from build123d import *

# Parameters (mm, degrees)
SKETCH_2_R = 0.5


with BuildPart() as part:
    # 扫描1: sweep along a path in 草图1
    with BuildLine(Plane.XY) as sweep_1_path:
        Line((-0.5, 0), (-4, 0))
        Line((-4, 0), (-4, 2))
        ThreePointArc((-4, 2), (0, 6), (4, 2))
        Line((4, 2), (4, 0))
        Line((4, 0), (0.5, 0))
    # 草图2 → 扫描1 (sweep)
    with BuildSketch(Plane(origin=(-0.5, 0, 0), x_dir=(0, 0, -1), z_dir=(1, 0, 0))):
        Circle(SKETCH_2_R)
    sweep(path=sweep_1_path.line, transition=Transition.RIGHT)


solid = part.part
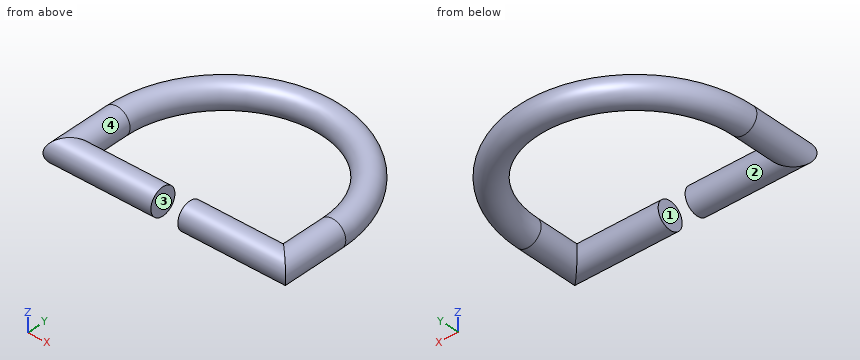
CAD build for the part. Positions are in the model's coordinates, mm. Face numbers are marked on the shaded views. A direction names the side the tool comes from. Coordinates: 2 decimals unless noted, no trailing zeros. Order: outer loops, then holes, each group sorted by start corner. A loop starts at its lowest first (then second) coordinate and runs counter-clockwise, first axis right, second up.
Item 1: 3-axis set-ups, long thin cutter, end or side, ignore diameter. For the marked faces 1 and 2: which of +Z, -Z, +X, -X, +Y, -Y reach the whole face in a straight line?
Check sheet entries:
face 1: +Z, -Z, -Y
face 2: none
Item 2: Two-plate mould, pull along Y, no slides. Class the marked faces 3 and 4: +Y half, -Y half, draft (parallel to the pull), parting line (faces both ways), or undercut.
Check sheet entries:
face 3: draft
face 4: undercut
Item 3: Drill centre lines: L1, parallel to Z at x = -2, y = 5.5; L2, parallel to Y at x = -1.25, z = -0.1; L3, parallel to Y at x = 1.75, z = -0.1. Where is each one in solid material? Low to high.
Check sheet entries:
L1: z = -0.5 to 0.5
L2: y = -0.49 to 0.49, 5.28 to 6.31
L3: y = -0.49 to 0.49, 5.04 to 6.13
Item 4: Band-saw the part on C-C on y = 1.25. List the corners of the cut face in (x, z).
Check sheet entries:
outline: circle Ø1 at (-4, 0); circle Ø1 at (4, 0)
Item 5: Band-saw the part on A-A on y = 0. List the corners of the cut face in (x, z).
Check sheet entries:
outline: (-4, -0.5) - (-0.5, -0.5) - (-0.5, 0.5) - (-4, 0.5) arc R0.5 ccw to start; (0.5, -0.5) - (4, -0.5) arc R0.5 ccw to (4, 0.5) - (0.5, 0.5) - close
Item 6: Band-saw the part on B-B on z = -0.3. List the corners of the cut face in (x, y), plus the area to 3 significant figures.
Check sheet entries:
outline: (-4.4, -0.4) - (-0.5, -0.4) - (-0.5, 0.4) - (-3.6, 0.4) - (-3.6, 2) arc R3.6 cw to (3.6, 2) - (3.6, 0.4) - (0.5, 0.4) - (0.5, -0.4) - (4.4, -0.4) - (4.4, 2) arc R4.4 ccw to (-4.4, 2) - close
area: 18.9 mm2
Item 7: Pin check, flat tip, straight feed: pin 1 Ø1 at (x, y) = (-1, 0.5) entering from -Z. Stop position of the tip, or through.
Check sheet entries:
pin 1: stops at z = -0.5
